```python
from build123d import *
from build123d.topology import SkipClean

# Parameters (mm, degrees)
SKETCH1_W               = 195
SKETCH1_H               = 136
SKETCH1_W_2             = 171
SKETCH1_H_2             = 112
SKETCH1_W_3             = 160
SKETCH1_H_3             = 96
SKETCH1_W_4             = 29
SKETCH1_H_4             = 3
BOSS_EXTRUDE1_DEPTH     = 2
SKETCH1_3_W             = 195
SKETCH1_3_H             = 136
BOSS_EXTRUDE2_DEPTH     = 2
CUT_EXTRUDE1_DEPTH      = 1.375
CUT_EXTRUDE1_DEPTH_BACK = 1.375
SKETCH2_R               = 3.25
SKETCH3_R               = 19.314272249
CUT_EXTRUDE2_DEPTH      = 119.938009064
SKETCH5_W               = 20
SKETCH5_H               = 3
SKETCH5_W_2             = 3
SKETCH5_H_2             = 10
BOSS_EXTRUDE3_DEPTH     = 3
CUT_EXTRUDE3_DEPTH      = 184.163861064
CUT_EXTRUDE4_DEPTH      = 152.615467549


with BuildPart() as part:
    # Sketch1 → Boss-Extrude1 (new body)
    # profile 1 of 3: a face of its own
    with BuildSketch(Plane.XY):
        Rectangle(SKETCH1_W, SKETCH1_H)
        Polygon((85.5, 56), (85.5, -56), (14.5, -56), (14.5, -59), (-14.5, -59), (-14.5, -56), (-85.5, -56), (-85.5, 56), align=None, mode=Mode.SUBTRACT)
    # profile 2 of 3: a face of its own
    with BuildSketch(Plane.XY):
        Rectangle(SKETCH1_W_2, SKETCH1_H_2)
        with Locations((0, 3)):
            Rectangle(SKETCH1_W_3, SKETCH1_H_3, mode=Mode.SUBTRACT)
    # profile 3 of 3: a face of its own
    with BuildSketch(Plane.XY):
        with Locations((0, -57.5)):
            Rectangle(SKETCH1_W_4, SKETCH1_H_4)
    extrude(amount=-BOSS_EXTRUDE1_DEPTH)

    # Sketch1_3 → Boss-Extrude2 (add)
    with BuildSketch(Plane.XY):
        Rectangle(SKETCH1_3_W, SKETCH1_3_H)
        Polygon((85.5, 56), (85.5, -56), (14.5, -56), (14.5, -59), (-14.5, -59), (-14.5, -56), (-85.5, -56), (-85.5, 56), align=None, mode=Mode.SUBTRACT)
    extrude(amount=BOSS_EXTRUDE2_DEPTH)

    # Sketch2 → Cut-Extrude1 (cut, two sides: drawn at the far end of the back side and taken through both)
    with SkipClean():  # the faces are left unmerged after this step: merging them gives an invalid solid
        with BuildSketch(Plane.XY.offset(-CUT_EXTRUDE1_DEPTH_BACK)):
            with Locations((-90.5, 61)):
                Circle(SKETCH2_R)
            with Locations((90.5, 61)):
                Circle(SKETCH2_R)
            with Locations((90.5, -61)):
                Circle(SKETCH2_R)
            with Locations((-90.5, -61)):
                Circle(SKETCH2_R)
            with Locations((-30.166666667, -61)):
                Circle(SKETCH2_R)
            with Locations((30.166666667, -61)):
                Circle(SKETCH2_R)
            with Locations((90.5, 0)):
                Circle(SKETCH2_R)
            with Locations((-30.166666667, 61)):
                Circle(SKETCH2_R)
            with Locations((30.166666667, 61)):
                Circle(SKETCH2_R)
            with Locations((-90.5, 0)):
                Circle(SKETCH2_R)
        extrude(amount=CUT_EXTRUDE1_DEPTH + CUT_EXTRUDE1_DEPTH_BACK, mode=Mode.SUBTRACT)

    # Sketch3 → Cut-Extrude2 (cut, through all)
    with SkipClean():  # the faces are left unmerged after this step: merging them gives an invalid solid
        with BuildSketch(Plane(origin=(0, 0, -2), x_dir=(-1, 0, 0), z_dir=(0, 0, -1))):
            with Locations((97.5, -68)):
                Circle(SKETCH3_R)
        cut_extrude2 = extrude(amount=-CUT_EXTRUDE2_DEPTH, mode=Mode.SUBTRACT)

    # Mirror1: Cut-Extrude2 across plane
    with SkipClean():  # the faces are left unmerged after this step: merging them gives an invalid solid
        add(cut_extrude2.mirror(Plane(origin=(0, 0, 0), x_dir=(0, 0, 1), z_dir=(1, 0, 0))), mode=Mode.SUBTRACT)

    # Sketch5 → Boss-Extrude3 (add)
    with SkipClean():  # the faces are left unmerged after this step: merging them gives an invalid solid
        with BuildSketch(Plane.XY.offset(2)):
            with Locations((-62.5, -66.5)):
                Rectangle(SKETCH5_W, SKETCH5_H)
            with Locations((62.5, -66.5)):
                Rectangle(SKETCH5_W, SKETCH5_H)
            with Locations((-96, 43)):
                Rectangle(SKETCH5_W_2, SKETCH5_H_2)
            with Locations((96, 43)):
                Rectangle(SKETCH5_W_2, SKETCH5_H_2)
        extrude(amount=BOSS_EXTRUDE3_DEPTH)

    # Sketch6 → Cut-Extrude3 (cut, through all)
    with SkipClean():  # the faces are left unmerged after this step: merging them gives an invalid solid
        with BuildSketch(Plane(origin=(72.5, 0, 0), x_dir=(0, 0, -1), z_dir=(1, 0, 0))):
            Polygon((-3.5, -66), (-5, -65), (-2, -65), align=None)
        extrude(amount=-CUT_EXTRUDE3_DEPTH, mode=Mode.SUBTRACT)

    # Sketch7 → Cut-Extrude4 (cut, through all)
    with SkipClean():  # the faces are left unmerged after this step: merging them gives an invalid solid
        with BuildSketch(Plane(origin=(0, 48, 0), x_dir=(1, 0, 0), z_dir=(0, 1, 0))):
            Polygon((94.5, -2), (95.5, -3.5), (94.5, -5), align=None)
        cut_extrude4 = extrude(amount=-CUT_EXTRUDE4_DEPTH, mode=Mode.SUBTRACT)

    # Mirror2: Cut-Extrude4 across plane
    with SkipClean():  # the faces are left unmerged after this step: merging them gives an invalid solid
        add(cut_extrude4.mirror(Plane(origin=(0, 0, 0), x_dir=(0, 0, 1), z_dir=(1, 0, 0))), mode=Mode.SUBTRACT)


solid = part.part
```
Can you work these out from the model? Positions are in its coordinate system, mm. A direction names the side the tool comes from. Coordinates: 2 decimals unless noted, no trailing zeros. Loops run counter-clockwise (first coordinate to the right, second up) from the corner with the lowest first, then second, coordinate; pieces in that order, holes last.
Item 1: Which directions (+Z, -Z, +X, -X, +Y, -Y) give clear straight access to the entire face, cutting with the end or side of a thin tool? Please do faces 3 (the face through (30, -61, -1.375)), 4 (the face through (97.5, 9, 0)).
Answers below:
face 3: none
face 4: +Z, -Z, +X, +Y, -Y
Item 2: I'm going to push flat-ended pins straight in: pin 1 (0.9 mm diameter, centred on y = -67, z = 3.5, fed in from +X); pin 2 (0.6 mm diameter, centred on y = -57, z = 1, fed in from -X); pin 3 (3.5 mm diameter, centred on y = -66.5, z = 3, fed in from -X); pin 4 (10 mm diameter, centred on x = -9.5, y = -43.5, fed in from -Z). Where does each tip first touch, or does it pass through?
Answers below:
pin 1: stops at x = 72.5
pin 2: stops at x = -81.84
pin 3: stops at x = -78.41
pin 4: stops at z = -2
Item 3: Suppose I cut it at B-B (x = 4). Please give me the cut outline in (y, z).
Answers below:
outline: (-68, -2) - (-45, -2) - (-45, 0) - (-59, 0) - (-59, 2) - (-68, 2) - close; (51, -2) - (68, -2) - (68, 2) - (56, 2) - (56, 0) - (51, 0) - close
Item 4: Suppose I cut it at C-C (y = -16). Please give me the cut outline in (x, z).
Answers below:
outline: (-97.5, -2) - (-80, -2) - (-80, 0) - (-85.5, 0) - (-85.5, 2) - (-97.5, 2) - close; (80, -2) - (97.5, -2) - (97.5, 2) - (85.5, 2) - (85.5, 0) - (80, 0) - close
Item 5: Suppose I cut it at A-A (y = 0). Please give me the cut outline in (x, z) (3 decimals), then the cut area to 4 significant figures.
Answers below:
outline: (-97.5, -2) - (-80, -2) - (-80, 0) - (-85.5, 0) - (-85.5, 2) - (-97.5, 2) - close; (80, -2) - (97.5, -2) - (97.5, 2) - (85.5, 2) - (85.5, 0) - (80, 0) - close; hole (-93.75, -1.375) - (-87.25, -1.375) - (-87.25, 1.375) - (-93.75, 1.375) - close; hole (87.25, -1.375) - (93.75, -1.375) - (93.75, 1.375) - (87.25, 1.375) - close
area: 82.25 mm2
Item 6: Suppose I cut it at D-D (y = 61). Please give me the cut outline in (x, z) (3 decimals), then the cut area to 4 significant figures.
Answers below:
outline: (-97.5, -2) - (97.5, -2) - (97.5, 2) - (-97.5, 2) - close; hole (-93.75, -1.375) - (-87.25, -1.375) - (-87.25, 1.375) - (-93.75, 1.375) - close; hole (-33.417, -1.375) - (-26.917, -1.375) - (-26.917, 1.375) - (-33.417, 1.375) - close; hole (26.917, -1.375) - (33.417, -1.375) - (33.417, 1.375) - (26.917, 1.375) - close; hole (87.25, -1.375) - (93.75, -1.375) - (93.75, 1.375) - (87.25, 1.375) - close
area: 708.5 mm2
Item 7: Please list where these lines run through material, in increasing order: L1, parallel to Y at x = 19.5, z = 1.5; L2, parallel to X at y = 22, z = -0.5; L3, parallel to X at y = -11.5, z = 1.25.
Answers below:
L1: y = -68 to -56, 56 to 68
L2: x = -97.5 to -80, 80 to 97.5
L3: x = -97.5 to -85.5, 85.5 to 97.5
Item 8: If we mould it in two halves opening along Z, with no side actions, what happens to faces 1 (the face through (-97.5, 9, 0)), 2 (the face through (90, 61, -1.375))? For each: released by +Z, released by -Z, zero draft, split by the parting line, or undercut.
Answers below:
face 1: zero draft
face 2: undercut
